Source: CAD feature listing. Evaluate the final solid. Frame: model axes, mm. Face numbers are marked on the shaded views. A direction names the side the tool comes from. Coordinates: 2 decimals unless noted, no trailing zeros. Write each loop counter-clockwise with the first axis right and the second up, starting at its lowest first coordinate (ties: lowest second). Pieces come first, ordered by that corner, then holes. Notation, with made-up numbers: (55.5, 7) - (103.5, 7) arc R33 cw to (103.5, 46) - close; hole circle Ø8 at (59, 44.5). An arc over 180 degrees is marked (long way). One line per question, with ' | ' between items. Start each with the question number.
Q1. Cut plane C-C, the plane y = 13. Give the number of separate pieces and of enclosed holes in the cut face, plus the area to 3 significant figures.
Q2. Contact query for flat-ended pins moving along their axis: P1, Ø6, axis at x = 1.5, y = 7, coming from the +Z side; P2, Ø0.9, axis at x = -16, y = 13, coming from the -Z side; P3, Ø2, axis at x = -8.5, z = 2.5, coming from the +Y side. Output: stop coordinate, or through.
Q3. Access query for the marked faces 4, 5 and 6. Directions: +Z, -Z, +X, -X, +Y, -Y. A direction counts if a zero-diameter tool reaches every point of the face in a straight line with its end or side. Return the directions, or none.
Q4. Line query: line 1 (Z direction, x = -40.5, y = 16); line 2 (Z direction, x = -33, y = 10); line 3 (X direction, y = 14, z = 2.5). Output: solid intervals per line, ascending.
Q5. Cut plane B-B, the plane z = 29. Return loops of the section in (x, y).
Q6. Draft query along Z for the marked faces 1, 2 and 3. Return one class per face: +Z half, -Z half, draft (parallel to the pull), parting line (faces both ways), or undercut.
Q7. Cut plane A-A, the plane x = -41.5. Return loops of the section in (y, z), plus the area to 3 significant figures.
Q8. Cut plane D-D, the plane x = -22. Return loops of the section in (y, z).
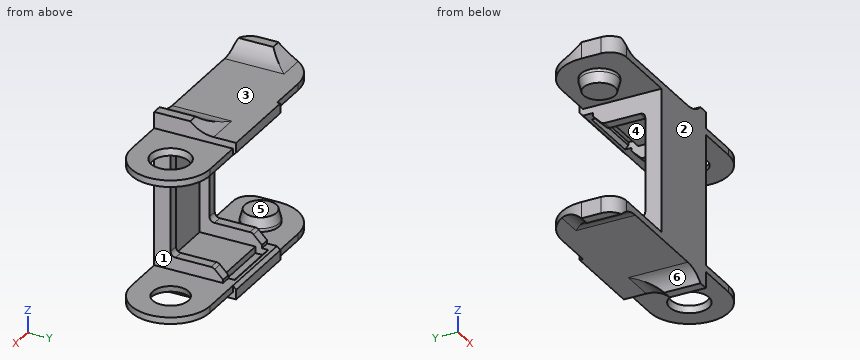
```python
from build123d import *

# Parameters (mm, degrees)
SKETCH_1_W             = 25
SKETCH_1_H             = 25
EXTRUDE_1_DEPTH        = 4
SKETCH_2_W             = 25
SKETCH_2_H             = 24
EXTRUDE_2_DEPTH        = 2
SKETCH_3_R             = 5.625
EXTRUDE_3_DEPTH        = 4
CHAMFER_1_SIZE         = 3
CHAMFER_1_SIZE2        = 0.803847577
EXTRUDE_4_DEPTH        = 2
SKETCH_6_R             = 5
CUT_EXTRUDE_2_DEPTH    = 10
EXTRUDE_6_DEPTH        = 20
SKETCH_9_W             = 19
SKETCH_9_H             = 3
CUT_EXTRUDE_4_DEPTH    = 2
CHAMFER_2_SIZE         = 1
CHAMFER_3_SIZE         = 3.732050808
CHAMFER_3_SIZE_2       = 1
FILLET_1_R             = 13
CHAMFER_4_SIZE         = 1
SKETCH_11_W            = 3
SKETCH_11_H            = 4
EXTRUDE_7_DEPTH        = 16
PATTERN_LINEAR_1_COUNT = 2
PATTERN_LINEAR_1_PITCH = 22
CHAMFER_6_SIZE         = 3
FILLET_2_R             = 1.5
SKETCH1_W              = 3
SKETCH1_H              = 11
BOSS_EXTRUDE1_DEPTH    = 3
FILLET1_R              = 10
SKETCH2_W              = 3
SKETCH2_H              = 11
BOSS_EXTRUDE2_DEPTH    = 3
FILLET2_R              = 10
FILLET3_R              = 5


with BuildPart() as part:
    # Эскиз1 → Бобышка-Вытянуть1 (new body)
    with BuildSketch(Plane.XY):
        with Locations((-26.279531703, 11.219512195)):
            Rectangle(SKETCH_1_W, SKETCH_1_H)
    extrude(amount=EXTRUDE_1_DEPTH)

    # Эскиз2 → Бобышка-Вытянуть2 (add)
    with BuildSketch(Plane(origin=(0, 0, 0), x_dir=(-1, 0, 0), z_dir=(0, 0, -1))):
        with Locations((51.279531703, 10.719512195)):
            Rectangle(SKETCH_2_W, SKETCH_2_H)
    extrude(amount=-EXTRUDE_2_DEPTH)

    # Эскиз3 → Бобышка-Вытянуть3 (add)
    with BuildSketch(Plane.XY.offset(2)):
        with Locations((-51.779531703, 10.719512195)):
            Circle(SKETCH_3_R)
    extrude(amount=EXTRUDE_3_DEPTH)

    # Фаска1
    chamfer_1_edges = [part.edges().sort_by_distance(p)[0] for p in [
        (-57.404531703, 10.719512195, 6),
    ]]
    chamfer_1_side = [part.faces().sort_by_distance(p)[0] for p in [
        (-57.404531703, 10.719512195, 4),
    ]]
    chamfer(chamfer_1_edges, length=CHAMFER_1_SIZE, length2=CHAMFER_1_SIZE2, reference=chamfer_1_side[0])

    # Эскиз5 → Бобышка-Вытянуть4 (add)
    with BuildSketch(Plane.XY.offset(4)):
        with BuildLine():
            Line((-18.981970926, 22.719512195), (-0.779531703, 22.719512195))
            ThreePointArc((-0.779531703, 22.719512195), (11.220468297, 10.719512195), (-0.779531703, -1.280487805))
            Line((-0.779531703, -1.280487805), (-18.981970926, -1.280487805))
            ThreePointArc((-18.981970926, -1.280487805), (-30.981970926, 10.719512195), (-18.981970926, 22.719512195))
        make_face()
    extrude(amount=-EXTRUDE_4_DEPTH)

    # Эскиз6 → Вырез-Вытянуть2 (cut)
    with BuildSketch(Plane(origin=(0, 0, 2), x_dir=(-1, 0, 0), z_dir=(0, 0, -1))):
        with Locations((0.779531703, 10.719512195)):
            Circle(SKETCH_6_R)
    extrude(amount=-CUT_EXTRUDE_2_DEPTH, mode=Mode.SUBTRACT)

    # Эскиз8 → Бобышка-Вытянуть6 (add)
    with BuildSketch(Plane.XY.offset(4)):
        Polygon((-38.779531703, 3.719512195), (-35.779531703, 3.719512195), (-35.779531703, 0.719512195), (-16.779531703, 0.719512195), (-16.779531703, 3.719512195), (-13.779531703, 3.719512195), (-13.779531703, -1.280487805), (-38.779531703, -1.280487805), align=None)
    extrude(amount=EXTRUDE_6_DEPTH)

    # Эскиз9 → Вырез-Вытянуть4 (cut)
    with BuildSketch(Plane.XY.offset(4)):
        with Locations((-26.279531703, 19.219512195)):
            Rectangle(SKETCH_9_W, SKETCH_9_H)
    extrude(amount=-CUT_EXTRUDE_4_DEPTH, mode=Mode.SUBTRACT)

    # Фаска2
    chamfer_2_edges = [part.edges().sort_by_distance(p)[0] for p in [
        (-26.279531703, 20.719512195, 4),
    ]]
    chamfer(chamfer_2_edges, length=CHAMFER_2_SIZE)

    # Фаска3
    # the kernel refuses this chamfer: 3.732050808, 1 mm, written as the material it takes off along each edge
    with BuildSketch(Plane(origin=(-0.779531703, 10.719512195, 2), x_dir=(-1, 0, 0), z_dir=(0, -1, 0))) as chamfer_3_piece_1:
        Polygon((5, -CHAMFER_3_SIZE), (5 + CHAMFER_3_SIZE_2, 0), (5, 0), align=None)
    revolve(axis=Axis((-0.779531703, 10.719512195, 2), (0, 0, -1)), mode=Mode.SUBTRACT)

    # Скругление1
    fillet_1_edges = [part.edges().sort_by_distance(p)[0] for p in [
        (-63.779531703, 22.719512195, 1),
    ]]
    fillet(fillet_1_edges, radius=FILLET_1_R)

    # Фаска4
    chamfer_4_edges = [part.edges().sort_by_distance(p)[0] for p in [
        (-26.279531703, 23.719512195, 4),
    ]]
    chamfer(chamfer_4_edges, length=CHAMFER_4_SIZE)

    # Эскиз11 → Бобышка-Вытянуть7 (add)
    with BuildSketch(Plane(origin=(0, 3.719512195, 0), x_dir=(1, 0, 0), z_dir=(0, 1, 0))):
        with Locations((-37.279531703, -6)):
            Rectangle(SKETCH_11_W, SKETCH_11_H)
    extrude_7 = extrude(amount=EXTRUDE_7_DEPTH)

    # Линейный массив1: Бобышка-Вытянуть7 ×2
    with Locations(*[(i * PATTERN_LINEAR_1_PITCH, 0, 0) for i in range(1, PATTERN_LINEAR_1_COUNT)]):
        add(extrude_7)

    # Фаска6
    chamfer_6_edges = [part.edges().sort_by_distance(p)[0] for p in [
        (-37.279531703, 19.719512195, 8),
        (-15.279531703, 19.719512195, 8),
    ]]
    chamfer(chamfer_6_edges, length=CHAMFER_6_SIZE)

    # Скругление2
    fillet_2_edges = [part.edges().sort_by_distance(p)[0] for p in [
        (-37.279531703, 3.719512195, 8),
        (-15.279531703, 3.719512195, 8),
        (-15.279531703, 16.719512195, 8),
        (-37.279531703, 16.719512195, 8),
    ]]
    fillet(fillet_2_edges, radius=FILLET_2_R)

    # Sketch1 → Boss-Extrude1 (add)
    with BuildSketch(Plane(origin=(0, 0, 0), x_dir=(-1, 0, 0), z_dir=(0, 0, -1))):
        with Locations((15.279531703, 4.219512195)):
            Rectangle(SKETCH1_W, SKETCH1_H)
    extrude(amount=BOSS_EXTRUDE1_DEPTH)

    # Fillet1
    # the kernel refuses this fillet: 10 mm, written as the material it adds along each edge
    with BuildSketch(Plane(origin=(-16.779531703, 9.719512195, 0), x_dir=(-1, 0, 0), z_dir=(0, -1, 0))) as fillet1_piece_1:
        with BuildLine():
            CenterArc((7.141428429, 10), FILLET1_R, 224.427004001, 45.572995999)
            Line((0, 3), (-0.142828569, 2.86))
            ThreePointArc((-0.142828569, 2.86), (-0.2, 1.5), (-0.2, 0))
            Line((-0.2, 0), (0, -0.2))
            Line((0, -0.2), (7.141428429, -0.2))
            Line((7.141428429, -0.2), (7.141428429, 0))
        make_face()
    extrude(amount=11)
    with BuildSketch(Plane(origin=(-13.779531703, 9.719512195, 0), x_dir=(0, 1, 0), z_dir=(-1, 0, 0))) as fillet1_piece_2:
        with BuildLine():
            CenterArc((7.141428429, 10), FILLET1_R, 224.427004001, 45.572995999)
            Line((0, 3), (-0.142828569, 2.86))
            ThreePointArc((-0.142828569, 2.86), (-0.2, 1.5), (-0.2, 0))
            Line((-0.2, 0), (0, -0.2))
            Line((0, -0.2), (7.141428429, -0.2))
            Line((7.141428429, -0.2), (7.141428429, 0))
        make_face()
    extrude(amount=3)
    with BuildSketch(Plane(origin=(-16.779531703, 27.573083266, 0), x_dir=(-1, 0, 0), z_dir=(0, -1, 0))) as fillet1_piece_3a_section:
        with BuildLine():
            CenterArc((7.141428429, 10), FILLET1_R, 224.427004001, 45.572995999)
            Line((0, 3), (-0.142828569, 2.86))
            ThreePointArc((-0.142828569, 2.86), (-0.2, 1.5), (-0.2, 0))
            Line((-0.2, 0), (0, -0.2))
            Line((0, -0.2), (7.141428429, -0.2))
            Line((7.141428429, -0.2), (7.141428429, 0))
        make_face()
    fillet1_piece_3a = extrude(amount=28.853571071, mode=Mode.PRIVATE)
    fillet1_piece_3a = split(fillet1_piece_3a, bisect_by=Plane(origin=(-16.779531703, 23.719512195, 0), z_dir=(0, -1, 0)), keep=Keep.TOP, mode=Mode.PRIVATE)
    fillet1_piece_3a = split(fillet1_piece_3a, bisect_by=Plane(origin=(-16.779531703, 9.719512195, 0), z_dir=(0, 1, 0)), keep=Keep.TOP, mode=Mode.PRIVATE)
    with BuildSketch(Plane(origin=(-13.779531703, 9.719512195, 0), x_dir=(0, 1, 0), z_dir=(-1, 0, 0))) as fillet1_piece_3b_section:
        with BuildLine():
            CenterArc((7.141428429, 10), FILLET1_R, 224.427004001, 45.572995999)
            Line((0, 3), (-0.142828569, 2.86))
            ThreePointArc((-0.142828569, 2.86), (-0.2, 1.5), (-0.2, 0))
            Line((-0.2, 0), (0, -0.2))
            Line((0, -0.2), (7.141428429, -0.2))
            Line((7.141428429, -0.2), (7.141428429, 0))
        make_face()
    fillet1_piece_3b = extrude(amount=20.853571071, mode=Mode.PRIVATE)
    fillet1_piece_3b = split(fillet1_piece_3b, bisect_by=Plane(origin=(-16.779531703, 9.719512195, 0), z_dir=(-1, 0, 0)), keep=Keep.TOP, mode=Mode.PRIVATE)
    fillet1_piece_3 = fillet1_piece_3a & fillet1_piece_3b
    add(fillet1_piece_3)

    # Sketch2 → Boss-Extrude2 (add)
    with BuildSketch(Plane(origin=(0, 0, 0), x_dir=(-1, 0, 0), z_dir=(0, 0, -1))):
        with Locations((62.279531703, 4.219512195)):
            Rectangle(SKETCH2_W, SKETCH2_H)
    extrude(amount=BOSS_EXTRUDE2_DEPTH)

    # Fillet2
    # the kernel refuses this fillet: 10 mm, written as the material it adds along each edge
    with BuildSketch(Plane(origin=(-60.779531703, 9.719512195, 0), x_dir=(0, 1, 0), z_dir=(-1, 0, 0))) as fillet2_piece_1_section:
        with BuildLine():
            CenterArc((7.141428429, 10), FILLET2_R, 224.427004001, 45.572995999)
            Line((0, 3), (0, 0))
            Line((0, 0), (7.141428429, 0))
        make_face()
    fillet2_piece_1 = extrude(amount=20.853571071, mode=Mode.PRIVATE)
    fillet2_piece_1 = fillet2_piece_1 & Plane(origin=(-50.779531703, 9.719512195, 0), x_dir=(0, 1, 0), z_dir=(0, 0, 1)) * Cylinder(13, 71, mode=Mode.PRIVATE)
    add(fillet2_piece_1)
    with BuildSketch(Plane(origin=(-60.779531703, -1.280487805, 0), x_dir=(1, 0, 0), z_dir=(0, 1, 0))) as fillet2_piece_2:
        with BuildLine():
            CenterArc((7.141428429, 10), FILLET2_R, 224.427004001, 45.572995999)
            Line((0, 3), (0, 0))
            Line((0, 0), (7.141428429, 0))
        make_face()
    extrude(amount=11)
    with BuildSketch(Plane(origin=(-42.925960632, 9.719512195, 0), x_dir=(0, 1, 0), z_dir=(-1, 0, 0))) as fillet2_piece_3a_section:
        with BuildLine():
            CenterArc((7.141428429, 10), FILLET2_R, 224.427004001, 45.572995999)
            Line((0, 3), (0, 0))
            Line((0, 0), (7.141428429, 0))
        make_face()
    fillet2_piece_3a = extrude(amount=20.853571071, mode=Mode.PRIVATE)
    fillet2_piece_3a = split(fillet2_piece_3a, bisect_by=Plane(origin=(-60.779531703, 9.719512195, 0), z_dir=(1, 0, 0)), keep=Keep.TOP, mode=Mode.PRIVATE)
    with BuildSketch(Plane(origin=(-60.779531703, -1.280487805, 0), x_dir=(1, 0, 0), z_dir=(0, 1, 0))) as fillet2_piece_3b_section:
        with BuildLine():
            CenterArc((7.141428429, 10), FILLET2_R, 224.427004001, 45.572995999)
            Line((0, 3), (0, 0))
            Line((0, 0), (7.141428429, 0))
        make_face()
    fillet2_piece_3b = extrude(amount=28.853571071, mode=Mode.PRIVATE)
    fillet2_piece_3b = fillet2_piece_3b & Plane(origin=(-50.779531703, 9.719512195, 0), x_dir=(0, 1, 0), z_dir=(0, 0, 1)) * Cylinder(13, 87, mode=Mode.PRIVATE)
    fillet2_piece_3b = split(fillet2_piece_3b, bisect_by=Plane(origin=(-60.779531703, 9.719512195, 0), z_dir=(0, 1, 0)), keep=Keep.TOP, mode=Mode.PRIVATE)
    fillet2_piece_3 = fillet2_piece_3a & fillet2_piece_3b
    add(fillet2_piece_3)

    # Fillet3
    fillet3_edges = [part.edges().sort_by_distance(p)[0] for p in [
        (-63.779531703, -1.280487805, -0.5),
    ]]
    fillet(fillet3_edges, radius=FILLET3_R)

    # Зеркальное отражение1: part across plane


with BuildPart() as part_1:
    add(part.part)
    add(part.part.mirror(Plane(origin=(0, 0, 24), x_dir=(1, 0, 0), z_dir=(0, 0, -1))))


solid = part_1.part
```
Reply:
1) separate pieces: 4 | enclosed holes: 0 | area: 503 mm^2
2) P1: stops at z = 46 | P2: stops at z = -0.98 | P3: stops at y = 22.72
3) face 4: +Y | face 5: -X, +Y, -Y | face 6: -Z, +Y, -Y
4) line 1: z = 0 to 2, 46 to 48 | line 2: z = 0 to 4, 44 to 48 | line 3: x = -56.35 to -47.21, -38.78 to -5.64, 4.08 to 10.76
5) outline: (-38.78, -1.28) - (-13.78, -1.28) - (-13.78, 3.72) - (-16.78, 3.72) - (-16.78, 0.72) - (-35.78, 0.72) - (-35.78, 3.72) - (-38.78, 3.72) - close
6) face 1: undercut | face 2: draft | face 3: +Z half
7) outline: (-1.28, 0) - (22.72, 0) - (22.72, 2) - (-1.28, 2) - close; (-1.28, 46) - (22.72, 46) - (22.72, 48) - (-1.28, 48) - close | area: 96.0 mm^2
8) outline: (-1.28, -0.19) - (14.94, -0.19) arc R10 cw to (16.86, 0) - (23.72, 0) - (23.72, 3) - (22.72, 4) - (21.72, 4) - (20.72, 3) - (20.72, 2) - (17.72, 2) - (17.72, 4) - (0.72, 4) - (0.72, 44) - (17.72, 44) - (17.72, 46) - (20.72, 46) - (20.72, 45) - (21.72, 44) - (22.72, 44) - (23.72, 45) - (23.72, 48) - (16.86, 48) arc R10 cw to (14.94, 48.19) - (-1.28, 48.19) - close
